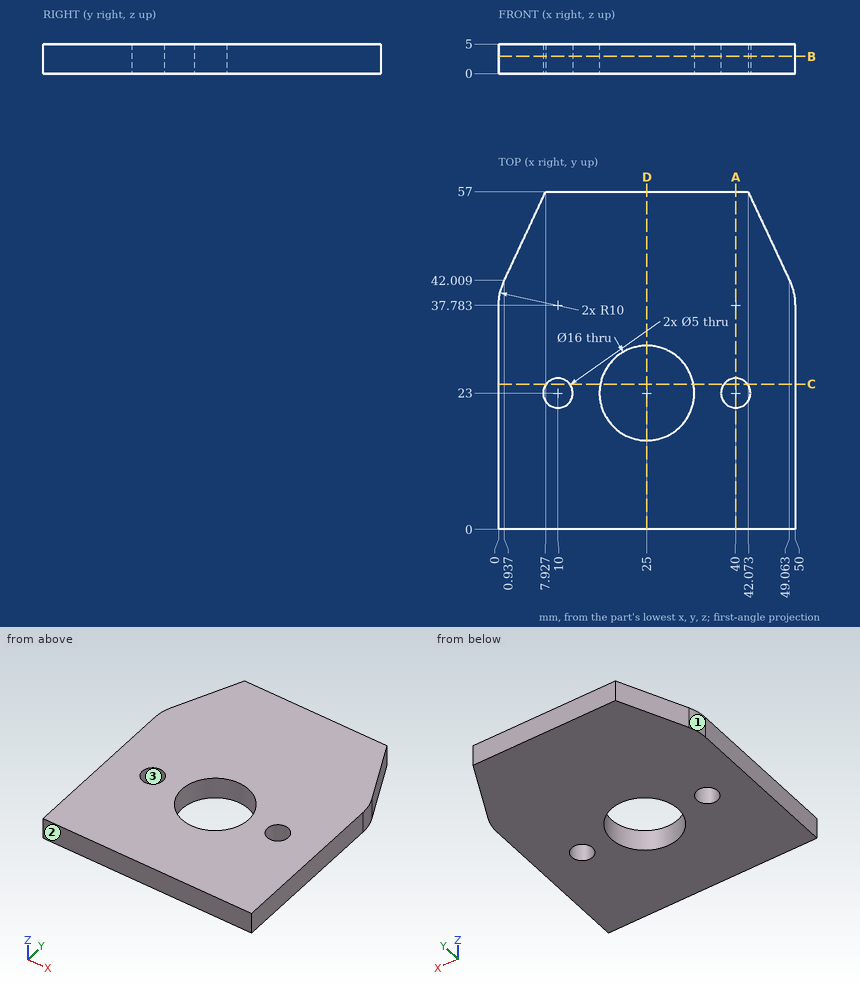
Study the drawing (mm; zero at the part's minimum x, y, z) and answer. Give positions to 0.01 mm unless a question says otherwise; leave off trailing zeros. Write each loop counter-clockwise with the first axis right and the second up, starting at its lowest first coordinate (ties: lowest second). Pieces come first, ordered by that corner, then holes. Notation, with made-up numbers: (26, 7.25) - (53, 7.25) arc R18 cw to (53, 14.25) - close; hole circle Ø11 at (-2.5, 15). An arc over 180 degrees is marked (long way). Use CSV: the item, a comma, the result in double quotes. Start each with the question number.
(1) Find section A-A (x = 40). Give the vertices of the cut face in (y, z).
(2) Find section D-D (x = 25). Give the vertices of the cut face in (y, z).
(3) Find section B-B (z = 2.9). Give the vertices of the cut face in (x, y), plus the area to 3 significant figures.
(4) Consider line 1 along Y through (x, z) = (40, 1.4); line 2 along Y through (x, z) = (25, 1.6); line 3 along X through (y, z) = (22, 2.8). Determine where each line is inside the solid, lowest interval first.
(5) Find section C-C (y = 24.5). Give the vertices of the cut face in (x, z), plus the area to 3 significant figures.
(6) Determine the mould class of the marked faces 1, 2 and 3 for opening direction X: +X half, -X half, draft (parallel to the pull), parting line (faces both ways), or undercut.
Findings below:
1,outline,"(0, 0) - (20.5, 0) - (20.5, 5) - (0, 5) - close; (25.5, 0) - (57, 0) - (57, 5) - (25.5, 5) - close"
2,outline,"(0, 0) - (15, 0) - (15, 5) - (0, 5) - close; (31, 0) - (57, 0) - (57, 5) - (31, 5) - close"
3,outline,"(0, 0) - (50, 0) - (50, 37.78) arc R10 ccw to (49.06, 42.01) - (42.07, 57) - (7.93, 57) - (0.94, 42.01) arc R10 ccw to (0, 37.78) - close; hole circle Ø5 at (10, 23); hole circle Ø16 at (25, 23); hole circle Ø5 at (40, 23)"
3,area,"2,470 mm2"
4,line 1,"0 to 20.5, 25.5 to 57"
4,line 2,"0 to 15, 31 to 57"
4,line 3,"0 to 7.71, 12.29 to 17.06, 32.94 to 37.71, 42.29 to 50"
5,outline,"(0, 0) - (8, 0) - (8, 5) - (0, 5) - close; (12, 0) - (17.14, 0) - (17.14, 5) - (12, 5) - close; (32.86, 0) - (38, 0) - (38, 5) - (32.86, 5) - close; (42, 0) - (50, 0) - (50, 5) - (42, 5) - close"
5,area,"131 mm2"
6,face 1,"-X half"
6,face 2,"draft"
6,face 3,"undercut"
